```python
from build123d import *

# Parameters (mm, degrees)
F0_W     = 80
F0_H     = 50
F1_DEPTH = 50
F2_W     = 60
F2_H     = 30
F3_DEPTH = 40
F4_R     = 15
F5_DEPTH = 10


with BuildPart() as f1:
    # F0 (on Top) → F1 (new body)
    with BuildSketch(Plane.XY):
        Rectangle(F0_W, F0_H)
    extrude(amount=F1_DEPTH)

    # F2 (on face) → F3 (cut)
    with BuildSketch(Plane.XY.offset(50)):
        Rectangle(F2_W, F2_H)
    extrude(amount=-F3_DEPTH, mode=Mode.SUBTRACT)

    # F4 (on face) → F5 (cut, through all)
    with BuildSketch(Plane.XZ.offset(25)):
        with Locations((10, 20)):
            Circle(F4_R)
    extrude(amount=-F5_DEPTH, mode=Mode.SUBTRACT)


solid = f1.part
```
Read the model definition and answer for the solid it produces. Units are mm, in the model's axes. A direction names the side the tool comes from. Round coordinates to 2 decimals unless told otherwise and drop trailing zeros. Write each loop counter-clockwise with the first axis right and the second up, starting at its lowest first coordinate (ties: lowest second). Pieces come first, ordered by that corner, then holes. Notation, with made-up numbers: (-3.75, -34) - (23.25, -34) arc R17 cw to (23.25, -6) - close; hole circle Ø10 at (56, 8.25). An arc over 180 degrees is marked (long way). Use CSV: the item, a comma, the result in double quotes.
Q1. A tool of negligible diameter and unlimited length cuts with its end or side. For faces 5 (the flat face through (40, 0, 25)), 6 (the cylindrical face through (6.748, -20.07, 5.357)), 7 (the flat face through (-30, 0, 30)), from which of +Z, -Z, +X, -X, +Y, -Y can it reach the whole face along a straight path? Write none if from no direction.
Values:
face 5,"+Z, -Z, +X, +Y, -Y"
face 6,"-Y"
face 7,"+Z"
Q2. Find section C-C, the plane z = 30.5. Write down the section's boundary in (x, y).
Values:
outline,"(-40, -25) - (-0.71, -25) - (-0.71, -15) - (-30, -15) - (-30, 15) - (30, 15) - (30, -15) - (20.71, -15) - (20.71, -25) - (40, -25) - (40, 25) - (-40, 25) - close"
Q3. Find section A-A, the plane x = 10. Write down the section's boundary in (y, z), then the cut area to 3 significant figures.
Values:
outline,"(-25, 0) - (25, 0) - (25, 50) - (15, 50) - (15, 10) - (-15, 10) - (-15, 5) - (-25, 5) - close; (-25, 35) - (-15, 35) - (-15, 50) - (-25, 50) - close"
area,"1,000 mm²"
Q4. Straight lines are drawn through the part: line 1 along X through (y, z) = (-21.5, 20); line 2 along Z through (x, y) = (10, -17); line 3 along Y through (x, z) = (-27, 28.5). For each, find the intervals that lie inside material, in ascending order.
Values:
line 1,"x = -40 to -5, 25 to 40"
line 2,"z = 0 to 5, 35 to 50"
line 3,"y = -25 to -15, 15 to 25"
Q5. Determine the mould class of faces 1 (the flat face through (-1, 17, 50)), 2 (the flat face through (10, -15, 8)), 3 (the flat face through (-1, 0, 0)), 4 (the flat face through (-9, -25, 25)) for opening direction Z: +Z half, -Z half, draft (parallel to the pull), parting line (faces both ways), or undercut.
Values:
face 1,"+Z half"
face 2,"undercut"
face 3,"-Z half"
face 4,"draft"
Q6. Each of these flat-tipped pins is pushed along its axis until it touches: pin 1 Ø1 at (x, y) = (21.5, 13) entering from +Z; pin 2 Ø18 at (x, z) = (10, 20) entering from -Y. Where does it stop, or does it pass through?
Values:
pin 1,"stops at z = 10"
pin 2,"stops at y = 15"
Q7. Find section D-D, the plane y = 0.5. Write down the section's boundary in (x, z).
Values:
outline,"(-40, 0) - (40, 0) - (40, 50) - (30, 50) - (30, 10) - (-30, 10) - (-30, 50) - (-40, 50) - close"
Q8. Find section B-B, the plane y = -17. Write down the section's boundary in (x, z), then the cut area to 3 significant figures.
Values:
outline,"(-40, 0) - (40, 0) - (40, 50) - (-40, 50) - close; hole circle Ø30 at (10, 20)"
area,"3,290 mm²"
